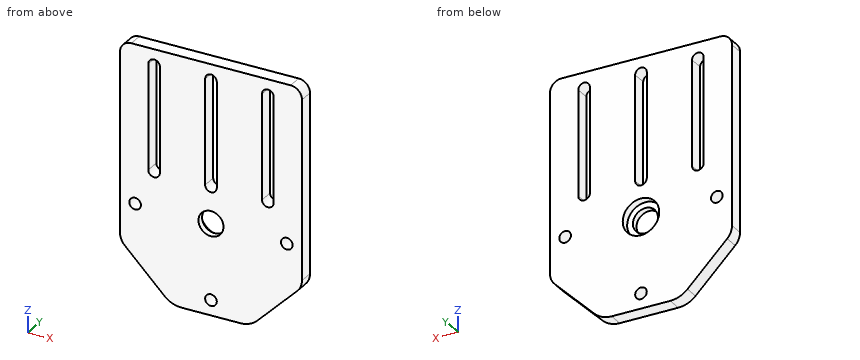
```python
from build123d import *

# Parameters (mm, degrees)
SKETCH1_R           = 5.5
SKETCH1_R_2         = 2.55
BOSS_EXTRUDE1_DEPTH = 6.35
SKETCH2_R           = 8.025
CUT_EXTRUDE1_DEPTH  = 3.5


with BuildPart() as part:
    # Sketch1 → Boss-Extrude1 (new body)
    with BuildSketch(Plane(origin=(0, 0, 0), x_dir=(1, 0, 0), z_dir=(0, 1, 0))):
        with BuildLine():
            Line((40, -27.5), (40, 14.306951673))
            ThreePointArc((40, 14.306951673), (39.448126611, 17.081406557), (37.876524164, 19.433475836))
            Line((37.876524164, 19.433475836), (20.438099577, 36.871900423))
            ThreePointArc((20.438099577, 36.871900423), (16.973258212, 39.187033407), (12.886199154, 40))
            Line((12.886199154, 40), (-12.886199154, 40))
            ThreePointArc((-12.886199154, 40), (-16.973258212, 39.187033407), (-20.438099577, 36.871900423))
            Line((-20.438099577, 36.871900423), (-37.876524164, 19.433475836))
            ThreePointArc((-37.876524164, 19.433475836), (-39.448126611, 17.081406557), (-40, 14.306951673))
            Line((-40, 14.306951673), (-40, -27.5))
            Line((-40, -27.5), (-40, -64.5))
            ThreePointArc((-40, -64.5), (-38.535533906, -68.035533906), (-35, -69.5))
            Line((-35, -69.5), (35, -69.5))
            ThreePointArc((35, -69.5), (38.535533906, -68.035533906), (40, -64.5))
            Line((40, -64.5), (40, -27.5))
        make_face()
        with Locations(Location((0, 0, 0), (0, 0, 270))):
            Circle(SKETCH1_R, mode=Mode.SUBTRACT)
        with Locations(Location((-33.333013665, 0, 0), (0, 0, 270))):
            Circle(SKETCH1_R_2, mode=Mode.SUBTRACT)
        with Locations(Location((0, 33.333013665, 0), (0, 0, 270))):
            Circle(SKETCH1_R_2, mode=Mode.SUBTRACT)
        with Locations(Location((33.333013665, 0, 0), (0, 0, 90))):
            Circle(SKETCH1_R_2, mode=Mode.SUBTRACT)
        with BuildLine():
            Line((22.45, -62.5), (22.45, -16.25))
            ThreePointArc((22.45, -16.25), (25, -13.7), (27.55, -16.25))
            Line((27.55, -16.25), (27.55, -62.5))
            ThreePointArc((27.55, -62.5), (25, -65.05), (22.45, -62.5))
        make_face(mode=Mode.SUBTRACT)
        with BuildLine():
            Line((-2.55, -62.5), (-2.55, -16.25))
            ThreePointArc((-2.55, -16.25), (0, -13.7), (2.55, -16.25))
            Line((2.55, -16.25), (2.55, -62.5))
            ThreePointArc((2.55, -62.5), (0, -65.05), (-2.55, -62.5))
        make_face(mode=Mode.SUBTRACT)
        with BuildLine():
            Line((-27.55, -62.5), (-27.55, -16.25))
            ThreePointArc((-27.55, -16.25), (-25, -13.7), (-22.45, -16.25))
            Line((-22.45, -16.25), (-22.45, -62.5))
            ThreePointArc((-22.45, -62.5), (-25, -65.05), (-27.55, -62.5))
        make_face(mode=Mode.SUBTRACT)
    extrude(amount=BOSS_EXTRUDE1_DEPTH)

    # Sketch2 → Cut-Extrude1 (cut)
    with BuildSketch(Plane(origin=(0, 6.35, 0), x_dir=(1, 0, 0), z_dir=(0, 1, 0))):
        with Locations(Location((0, 0, 0), (0, 0, 270))):
            Circle(SKETCH2_R)
    extrude(amount=-CUT_EXTRUDE1_DEPTH, mode=Mode.SUBTRACT)


solid = part.part
```
Work out the finished part from the listing and answer in its coordinate system (mm). Give positions to 0.01 mm unless a question says otherwise; leave off trailing zeros. Loops run counter-clockwise (first coordinate to the right, second up) from the corner with the lowest first, then second, coordinate; pieces in that order, holes last. Notation, with made-up numbers: M 67.25,63.25 L 113.25,63.25 A26 ccw 113.25,99.25 Z; hole C -35,-0.5 d2. An arc over 180 degrees is marked long. One line per item, written item: value. Start each with the question number.
1. Find section D-D (y = 1.5). Give the vertices of the cut face in (x, z), and give its area (3 significant figures).
2. Each of these flat-tipped pins is pushed along its axis until it touches: P1, Ø5, axis at x = 2, z = -3.5, coming from the +Y side; P2, Ø3, axis at x = 23, y = 3, coming from the -Z side; P3, Ø3, axis at y = 5.5, z = -28.5, coming from the +X side. Where does it stop, or does it pass through?
3. Find section A-A (x = -25). Give the vertices of the cut face in (y, z), and give its area (3 significant figures).
4. Find section B-B (x = 0). Give the vertices of the cut face in (y, z) (3 decimals), and give its area (3 significant figures).
5. Find the intervals of material crossed by probe 1 along X at (y, z) = (4, 0) (3 decimals); probe 2 along X at (y, z) = (2, 60.5); probe 3 along X at (y, z) = (1.75, -14.5), in increasing order.
6. Find section C-C (z = 55). Give the vertices of the cut face in (x, y), and give its area (3 significant figures).
Reported:
1. outline: M -40,-14.31 A7.25 ccw -37.88,-19.43 L -20.44,-36.87 A10.68 ccw -12.89,-40 L 12.89,-40 A10.68 ccw 20.44,-36.87 L 37.88,-19.43 A7.25 ccw 40,-14.31 L 40,64.5 A5 ccw 35,69.5 L -35,69.5 A5 ccw -40,64.5 Z; hole C -33.33,0 d5.1; hole M -27.55,16.25 A2.55 ccw -22.45,16.25 L -22.45,62.5 A2.55 ccw -27.55,62.5 Z; hole C 0,0 d11; hole C 0,-33.33 d5.1; hole M -2.55,16.25 A2.55 ccw 2.55,16.25 L 2.55,62.5 A2.55 ccw -2.55,62.5 Z; hole M 22.45,16.25 A2.55 ccw 27.55,16.25 L 27.55,62.5 A2.55 ccw 22.45,62.5 Z; hole C 33.33,0 d5.1
1. area: 7,300 mm²
2. P1: stops at y = 2.85
2. P2: stops at z = -35.81
2. P3: stops at x = 30.31
3. outline: M 0,-32.31 L 6.35,-32.31 L 6.35,13.7 L 0,13.7 Z; M 0,65.05 L 6.35,65.05 L 6.35,69.5 L 0,69.5 Z
3. area: 320 mm²
4. outline: M 0,-40 L 6.35,-40 L 6.35,-35.883 L 0,-35.883 Z; M 0,-30.783 L 6.35,-30.783 L 6.35,-8.025 L 2.85,-8.025 L 2.85,-5.5 L 0,-5.5 Z; M 0,5.5 L 2.85,5.5 L 2.85,8.025 L 6.35,8.025 L 6.35,13.7 L 0,13.7 Z; M 0,65.05 L 6.35,65.05 L 6.35,69.5 L 0,69.5 Z
4. area: 249 mm²
5. probe 1: x = -40 to -35.883, -30.783 to -8.025, 8.025 to 30.783, 35.883 to 40
5. probe 2: x = -40 to -27.55, -22.45 to -2.55, 2.55 to 22.45, 27.55 to 40
5. probe 3: x = -40 to 40
6. outline: M -40,0 L -27.55,0 L -27.55,6.35 L -40,6.35 Z; M -22.45,0 L -2.55,0 L -2.55,6.35 L -22.45,6.35 Z; M 2.55,0 L 22.45,0 L 22.45,6.35 L 2.55,6.35 Z; M 27.55,0 L 40,0 L 40,6.35 L 27.55,6.35 Z
6. area: 411 mm²
